from build123d import *

# Parameters (mm, degrees)
F0_W     = 600
F0_H     = 12
F1_DEPTH = 500
F2_DEPTH = 12


with BuildPart() as f1:
    # F0 (on Top) → F1 (new body)
    with BuildSketch(Plane.XY):
        with Locations((-808.5126264931, 528.488914907)):
            Rectangle(F0_W, F0_H)
    extrude(amount=F1_DEPTH)



with BuildPart() as f1b:
    # F0 (on Top) → F1, piece 2 (new body)
    with BuildSketch(Plane.XY):
        with Locations((-808.5126264931, -659.511085093)):
            Rectangle(F0_W, F0_H)
    extrude(amount=F1_DEPTH)


with BuildPart() as f1_1:
    add(f1.part)

    add(f1b.part)  # F2 merges F1b
    # F0 (on Top) → F2 (join)
    with BuildSketch(Plane.XY):
        Polygon((-508.5126264931, 522.488914907), (-1108.5126264931, 522.488914907), (-1108.5126264931, -653.511085093), (-508.5126264931, -653.511085093), (-508.5126264931, -609.109044075), align=None)
    extrude(amount=F2_DEPTH)


solid = f1_1.part
Check sheet for the modelled part. Datum: model origin and axes. Units: mm. A direction names the side the tool comes from. Give positions to 0.01 mm unless a question says otherwise; leave off trailing zeros. Loops run counter-clockwise (first coordinate to the right, second up) from the corner with the lowest first, then second, coordinate; pieces in that order, holes last. Notation, with made-up numbers: M 44.25,69 L 64.25,69 A23 ccw 64.25,92 Z; hole C -0.5,48.25 d5. An arc over 180 degrees is marked long. Return JSON: item names as keys, results as strings. Group by question number.
1. Go/stop test with a flat-tipped pin: pin 1 (1.5 mm diameter, centred on x = -947, y = -68, fed in from +Z). Record where the tip stops, or that it passes through.
2. Mould release check, pull along Y, two halves, no side actions. Record for faces 3 (the flat face through (-813, 522.489, 253)), 4 (the flat face through (-813, -665.511, 246)), 5 (the flat face through (-1108.513, -63, 8)): released by +Y, released by -Y, zero draft, split by the parting line, or undercut.
3. Tool access check on faces 1 (the flat face through (-813, -57, 0)), 2 (the flat face through (-813, -57, 12)). Record the directions out of +Z, -Z, +X, -X, +Y, -Y that give a thin tool (end or side, any length) a straight path to the whole face; none if there is none.
4. Cross-section at C-C on y = 309. Record the boundary of the cut face in (x, z).
5. Cross-section at A-A on z = 151. Record the boundary of the cut face in (x, y), plus the area to 3 significant figures.
6. Cross-section at B-B on x = -982.5. Record the boundary of the cut face in (y, z), plus the area to 3 significant figures.
7. Thickness scan on L1, parallel to Y at x = -660.5, z = 101.5; L2, parallel to Z at x = -908.5, y = -144.5. Record the ranges inside material, lowest first.
Return value:
{
 "1": {"pin 1": "z = 12"},
 "2": {"face 3": "undercut", "face 4": "released by -Y", "face 5": "zero draft"},
 "3": {"face 1": "-Z, +X, -X, +Y, -Y", "face 2": "+Z, +X, -X"},
 "4": {"outline": "M -1108.51,0 L -508.51,0 L -508.51,12 L -1108.51,12 Z"},
 "5": {"outline": "M -1108.51,-665.51 L -508.51,-665.51 L -508.51,-653.51 L -1108.51,-653.51 Z; M -1108.51,522.49 L -508.51,522.49 L -508.51,534.49 L -1108.51,534.49 Z", "area": "14,400 mm^2"},
 "6": {"outline": "M -665.51,0 L 534.49,0 L 534.49,500 L 522.49,500 L 522.49,12 L -653.51,12 L -653.51,500 L -665.51,500 Z", "area": "26,100 mm^2"},
 "7": {"L1": "-665.51 to -653.51, 522.49 to 534.49", "L2": "0 to 12"}
}
